from build123d import *

# Parameters (mm, degrees)
F0_W     = 63.397132
F0_H     = 91.097686
F1_DEPTH = 25.4
F2_T     = -2.54
F3_R     = 2


with BuildPart() as f1:
    # F0 (on Top) → F1 (new body)
    with BuildSketch(Plane.XY):
        with Locations((-4.997522, 3.712451)):
            Rectangle(F0_W, F0_H)
    extrude(amount=F1_DEPTH)

    # F2
    f2_openings = [f1.faces().sort_by_distance(p)[0] for p in [
        (-4.997522, 3.712451, 25.4),
    ]]
    offset(amount=F2_T, openings=f2_openings)

    # F3
    f3_edges = [f1.edges().sort_by_distance(p)[0] for p in [
        (26.701044, 3.712451, 25.4),
        (-4.997522, -41.836392, 25.4),
        (-36.696088, 3.712451, 25.4),
        (-4.997522, 49.261294, 25.4),
    ]]
    fillet(f3_edges, radius=F3_R)


solid = f1.part
Part model, mm, in its own coordinate system. A direction names the side the tool comes from. Coordinates: 2 decimals unless noted, no trailing zeros. Loops run counter-clockwise (first coordinate to the right, second up) from the corner with the lowest first, then second, coordinate; pieces in that order, holes last. Notation, with made-up numbers: M 85.5,-8.5 L 106.5,-8.5 A25 cw 106.5,4.5 Z; hole C 37.5,-12 d7. An arc over 180 degrees is marked long. Use a Markdown table: item, result. Add a question column.
Q1. Mould opens along X. For faces 1 (the cylindrical face through (26.13, 4.35, 24.8)), 2 (the flat face through (-5, 46.721, 14)), 3 (the cylindrical face through (-36.126, 4.35, 24.799)) say: +X half, -X half, draft (parallel to the pull), parting line (faces both ways), or undercut.
Q2. Pin check, flat tip, straight feed: P1, Ø3, axis at x = 0.5, y = 17, coming from the +Z side. Stop position of the tip, or through.
Q3. Cut at B-B (z = 21.75). Write the cut outline in (x, y), and give its area (3 significant figures).
Q4. Which spindle directions (+Z, -Z, +X, -X, +Y, -Y) get a long thin tool onto all of the face, cutting with end or side? Do faces 4 (the flat face through (-5, -39.296, 14)), 5 (the flat face through (-5, -41.836, 12)). Say none if no direction does.
Q5. Cut at C-C (y = -24.5). Write the cut outline in (x, z).
Q6. Cut at A-A (x = -26). Write the cut outline in (y, z).
Q7. Probe L1, parallel to X at y = 13.5, z = 5.25; L2, parallel to Y at x = 10.5, z = 13.5; L3, parallel to Z at x = 9, y = 22.5. List the from-to ranges inside material, lowest first.
Worked out:
| question | item | result |
|---|---|---|
| 1 | face 1 | +X half |
| 1 | face 2 | undercut |
| 1 | face 3 | -X half |
| 2 | P1 | stops at z = 2.54 |
| 3 | outline | M -36.7,-41.84 L 26.7,-41.84 L 26.7,49.26 L -36.7,49.26 Z; hole M -34.16,-39.3 L 24.16,-39.3 L 24.16,46.72 L -34.16,46.72 Z |
| 3 | area | 759 mm2 |
| 4 | face 4 | +Z |
| 4 | face 5 | +Z, -Z, +X, -X, -Y |
| 5 | outline | M -36.7,0 L 26.7,0 L 26.7,23.4 A2 ccw 24.7,25.4 L 24.16,25.4 L 24.16,2.54 L -34.16,2.54 L -34.16,25.4 L -34.7,25.4 A2 ccw -36.7,23.4 Z |
| 6 | outline | M -41.84,0 L 49.26,0 L 49.26,23.4 A2 ccw 47.26,25.4 L 46.72,25.4 L 46.72,2.54 L -39.3,2.54 L -39.3,25.4 L -39.84,25.4 A2 ccw -41.84,23.4 Z |
| 7 | L1 | x = -36.7 to -34.16, 24.16 to 26.7 |
| 7 | L2 | y = -41.84 to -39.3, 46.72 to 49.26 |
| 7 | L3 | z = 0 to 2.54 |
